```python
from build123d import *

# Parameters (mm, degrees)
F1_DEPTH = 6.35
F2_R     = 0.8128


with BuildPart() as f1:
    # F0 (on Front) → F1 (new body)
    with BuildSketch(Plane.XZ):
        with BuildLine():
            ThreePointArc((-70.6882, 76.358423), (-71.801752, 75.897174), (-72.263, 74.783623))
            Line((-72.263, 74.783623), (-72.263, 65.458811))
            ThreePointArc((-72.263, 65.458811), (-71.801752, 64.34526), (-70.6882, 63.884011))
            Line((-70.6882, 63.884011), (-67.4878, 63.884011))
            ThreePointArc((-67.4878, 63.884011), (-62.7253, 59.121511), (-67.4878, 54.359011))
            Line((-67.4878, 54.359011), (-70.6882, 54.359011))
            ThreePointArc((-70.6882, 54.359011), (-71.801752, 53.897763), (-72.263, 52.784211))
            Line((-72.263, 52.784211), (-72.263, 26.064518))
            ThreePointArc((-72.263, 26.064518), (-71.801752, 24.950967), (-70.6882, 24.489718))
            Line((-70.6882, 24.489718), (-67.4878, 24.489718))
            ThreePointArc((-67.4878, 24.489718), (-62.7253, 19.727218), (-67.4878, 14.964718))
            Line((-67.4878, 14.964718), (-70.6882, 14.964718))
            ThreePointArc((-70.6882, 14.964718), (-71.801752, 14.50347), (-72.263, 13.389918))
            Line((-72.263, 13.389918), (-72.263, 5.860977))
            ThreePointArc((-72.263, 5.860977), (-71.801752, 4.747425), (-70.6882, 4.286177))
            Line((-70.6882, 4.286177), (0, 4.286177))
            Line((0, 4.286177), (70.6882, 4.286177))
            ThreePointArc((70.6882, 4.286177), (71.801752, 4.747425), (72.263, 5.860977))
            Line((72.263, 5.860977), (72.263, 13.389918))
            ThreePointArc((72.263, 13.389918), (71.801752, 14.50347), (70.6882, 14.964718))
            Line((70.6882, 14.964718), (67.4878, 14.964718))
            ThreePointArc((67.4878, 14.964718), (62.7253, 19.727218), (67.4878, 24.489718))
            Line((67.4878, 24.489718), (70.6882, 24.489718))
            ThreePointArc((70.6882, 24.489718), (71.801752, 24.950967), (72.263, 26.064518))
            Line((72.263, 26.064518), (72.263, 52.784211))
            ThreePointArc((72.263, 52.784211), (71.801752, 53.897763), (70.6882, 54.359011))
            Line((70.6882, 54.359011), (67.4878, 54.359011))
            ThreePointArc((67.4878, 54.359011), (62.7253, 59.121511), (67.4878, 63.884011))
            Line((67.4878, 63.884011), (70.6882, 63.884011))
            ThreePointArc((70.6882, 63.884011), (71.801752, 64.34526), (72.263, 65.458811))
            Line((72.263, 65.458811), (72.263, 74.783623))
            ThreePointArc((72.263, 74.783623), (71.801752, 75.897174), (70.6882, 76.358423))
            Line((70.6882, 76.358423), (3.71171, 76.358423))
            Line((3.71171, 76.358423), (-3.71171, 76.358423))
            Line((-3.71171, 76.358423), (-70.6882, 76.358423))
        make_face()
    extrude(amount=F1_DEPTH)

    # F2
    f2_edges = [f1.edges().sort_by_distance(p)[0] for p in [
        (-72.263, -6.35, 70.121217),
        (-71.801752, -6.35, 75.897174),
        (0, -6.35, 76.358423),
        (71.801752, -6.35, 75.897174),
        (72.263, -6.35, 70.121217),
        (71.801752, -6.35, 64.34526),
        (62.7253, -6.35, 59.121511),
        (69.088, -6.35, 63.884011),
        (69.088, -6.35, 54.359011),
        (71.801752, -6.35, 53.897763),
        (72.263, -6.35, 39.424365),
        (71.801752, -6.35, 24.950967),
        (69.088, -6.35, 24.489718),
        (62.7253, -6.35, 19.727218),
        (69.088, -6.35, 14.964718),
        (71.801752, -6.35, 14.50347),
        (72.263, -6.35, 9.625448),
        (71.801752, -6.35, 4.747425),
        (0, -6.35, 4.286177),
        (-71.801752, -6.35, 4.747425),
        (-72.263, -6.35, 9.625448),
        (-71.801752, -6.35, 14.50347),
        (-62.7253, -6.35, 19.727218),
        (-69.088, -6.35, 14.964718),
        (-69.088, -6.35, 24.489718),
        (-71.801752, -6.35, 24.950967),
        (-72.263, -6.35, 39.424365),
        (-71.801752, -6.35, 53.897763),
        (-62.7253, -6.35, 59.121511),
        (-69.088, -6.35, 54.359011),
        (-69.088, -6.35, 63.884011),
        (-71.801752, -6.35, 64.34526),
    ]]
    fillet(f2_edges, radius=F2_R)


solid = f1.part
```
Check sheet for the modelled part. Datum: model origin and axes. Units: mm. A direction names the side the tool comes from. Give positions to 0.01 mm unless a question says otherwise; leave off trailing zeros. One line per question, with ' | ' between items. Start each with the question number.
1. Set-up check for faces 1 (the flat face through (-1, -6.35, 41)), 2 (the flat face through (-69, -3, 24.49)), 3 (the flat face through (69, -3, 14.965)): record each of +Z, -Z, +X, -X, +Y, -Y from which the full face is reachable in a straight line by a thin tool's end or side.
2. Draft check along Z on faces 4 (the flat face through (72.263, -3, 39)), 5 (the flat face through (1, -3, 76.358)), 6 (the flat face through (-69, -3, 14.965)), 7 (the flat face through (-1, -3, 4.286)). Enter one of: released by +Z, released by -Z, zero draft, split by the parting line, or undercut.
3. Material ranges on line 1 along Z through (x, y) = (65.5, -1.5); line 2 along X through (y, z) = (-1.5, 19.5); line 3 along X through (y, z) = (-6, 32.5), recorded low to high. Write a range as [from, to].
Check result:
1) face 1: +Z, -Z, +X, -X, -Y | face 2: -X, +Y, -Y | face 3: +X, +Y, -Y
2) face 4: zero draft | face 5: released by +Z | face 6: undercut | face 7: released by -Z
3) line 1: z = [4.29, 15.4], [24.06, 54.79], [63.45, 76.36] | line 2: x = [-62.73, 62.73] | line 3: x = [-72.12, 72.12]
